from build123d import *

# Parameters (mm, degrees)
SKETCH1_W                                    = 120
SKETCH1_H                                    = 116
BOSS_EXTRUDE1_DEPTH                          = 9.525
CBORE_FOR_M4_HEX_HEAD_CAP_SCREW1_D           = 4.2
CBORE_FOR_M4_HEX_HEAD_CAP_SCREW1_CBORE_D     = 7.6
CBORE_FOR_M4_HEX_HEAD_CAP_SCREW1_CBORE_DEPTH = 4.5
SKETCH2_R                                    = 7
CUT_EXTRUDE1_DEPTH                           = 84.992414092
SKETCH5_R                                    = 1.65
CUT_EXTRUDE2_DEPTH                           = 10
SKETCH6_R                                    = 1.65
CUT_EXTRUDE3_DEPTH                           = 84.992414092
FILLET1_R                                    = 10


with BuildPart() as part:
    # Sketch1 → Boss-Extrude1 (new body)
    with BuildSketch(Plane.YZ):
        Rectangle(SKETCH1_W, SKETCH1_H)
    extrude(amount=BOSS_EXTRUDE1_DEPTH)

    # CBORE for M4 Hex Head Cap Screw1 (through all)
    with Locations(Plane(origin=(9.525, -15.556349186, 21.556349186), x_dir=(0, 0, 1), z_dir=(1, 0, 0))):
        with Locations((0, 0), (0, -31.112698372), (-31.112698372, -31.112698372), (-31.112698372, 0)):
            CounterBoreHole(CBORE_FOR_M4_HEX_HEAD_CAP_SCREW1_D / 2, CBORE_FOR_M4_HEX_HEAD_CAP_SCREW1_CBORE_D / 2, CBORE_FOR_M4_HEX_HEAD_CAP_SCREW1_CBORE_DEPTH)

    # Sketch2 → Cut-Extrude1 (cut, through all)
    with BuildSketch(Plane.YZ.offset(9.525)):
        with Locations(Location((0, 6, 0), (0, 0, 270))):
            Circle(SKETCH2_R)
    extrude(amount=-CUT_EXTRUDE1_DEPTH, mode=Mode.SUBTRACT)

    # Sketch5 → Cut-Extrude2 (cut)
    with BuildSketch(Plane(origin=(0, 0, -58), x_dir=(1, 0, 0), z_dir=(0, 0, -1))):
        with Locations(Location((4.7625, 27, 0), (0, 0, 180))):
            Circle(SKETCH5_R)
        with Locations(Location((4.7625, 0, 0), (0, 0, 180))):
            Circle(SKETCH5_R)
        with Locations(Location((4.7625, -27, 0), (0, 0, 180))):
            Circle(SKETCH5_R)
        with Locations(Location((4.7625, -54, 0), (0, 0, 180))):
            Circle(SKETCH5_R)
        with Locations(Location((4.7625, 54, 0), (0, 0, 180))):
            Circle(SKETCH5_R)
    extrude(amount=-CUT_EXTRUDE2_DEPTH, mode=Mode.SUBTRACT)

    # Sketch6 → Cut-Extrude3 (cut, through all)
    with BuildSketch(Plane.YZ.offset(9.525)):
        with Locations(Location((34, 40, 0), (0, 0, 270))):
            Circle(SKETCH6_R)
        with Locations(Location((34, -28, 0), (0, 0, 270))):
            Circle(SKETCH6_R)
        with Locations(Location((-34, -28, 0), (0, 0, 270))):
            Circle(SKETCH6_R)
        with Locations(Location((-34, 40, 0), (0, 0, 270))):
            Circle(SKETCH6_R)
    extrude(amount=-CUT_EXTRUDE3_DEPTH, mode=Mode.SUBTRACT)

    # Fillet1
    fillet1_edges = [part.edges().sort_by_distance(p)[0] for p in [
        (4.7625, -60, 58),
        (4.7625, 60, 58),
    ]]
    fillet(fillet1_edges, radius=FILLET1_R)


solid = part.part
CAD build for the part. Positions are in the model's coordinates, mm. A direction names the side the tool comes from. Give positions to 0.01 mm unless a question says otherwise; leave off trailing zeros. Loops run counter-clockwise (first coordinate to the right, second up) from the corner with the lowest first, then second, coordinate; pieces in that order, holes last. Notation, with made-up numbers: M 24.25,19 L 40.25,19 A9 cw 40.25,25 Z; hole C 71,70.5 d5. An arc over 180 degrees is marked long. Answer in a Markdown table with one row per item. Add a question column.
Item 1: Band-saw the part on A-A on y = 34. Give the cut face in (x, z) (3 decimals), then the cut area to 3 significant figures.
Item 2: Mould opens along X. For faces 1 (the face through (4.83, 56.99, 55.15)), 2 (the face through (4.977, -25.364, -53.07)), 3 (the face through (9.525, -1, 14)) say: +X half, -X half, draft (parallel to the pull), parting line (faces both ways), or undercut.
Item 3: Drop flat-ended pins along their axis: P1, Ø2, axis at x = 4.76, y = 27, coming from the -Z side; P2, Ø5.5, axis at x = 4.76, y = 54, coming from the +Z side. Give the stop position or say it passes through.
Item 4: Band-saw the part on B-B on z = -28. Give the cut face in (x, y) (3 decimals).
Item 5: Band-saw the part on C-C on y = 0. Give the cut face in (x, z) (1 decimal).
Item 6: Probe probe 1 along Y at (x, z) = (4, 6); probe 2 along Z at (x, y) = (4.5, -16); probe 3 along Y at (x, z) = (2.75, 39.5). List the from-to ranges inside material, lowest first.
Item 7: Tool access for faces 4 (the face through (4.977, 28.636, -53.07)), 5 (the face through (7.306, -13.244, 18.541)), 6 (the face through (2.477, 13.474, -9.283)): list every direction of +Z, -Z, +X, -X, +Y, -Y with a clear straight run to the whole face (end or side of a thin tool).
Item 8: Band-saw the part on D-D on y = -27. Give the cut face in (x, z) (1 decimal).
Reply:
| question | item | result |
|---|---|---|
| 1 | outline | M 0,-58 L 9.525,-58 L 9.525,-29.65 L 0,-29.65 Z; M 0,-26.35 L 9.525,-26.35 L 9.525,38.35 L 0,38.35 Z; M 0,41.65 L 9.525,41.65 L 9.525,58 L 0,58 Z |
| 1 | area | 1,040 mm^2 |
| 2 | face 1 | draft |
| 2 | face 2 | undercut |
| 2 | face 3 | +X half |
| 3 | P1 | stops at z = -48 |
| 3 | P2 | stops at z = 57.92 |
| 4 | outline | M 0,-60 L 9.525,-60 L 9.525,-35.65 L 0,-35.65 Z; M 0,-32.35 L 9.525,-32.35 L 9.525,32.35 L 0,32.35 Z; M 0,35.65 L 9.525,35.65 L 9.525,60 L 0,60 Z |
| 5 | outline | M 0,-58 L 3.1,-58 L 3.1,-48 L 6.4,-48 L 6.4,-58 L 9.5,-58 L 9.5,-1 L 0,-1 Z; M 0,13 L 9.5,13 L 9.5,58 L 0,58 Z |
| 6 | probe 1 | y = -60 to -7, 7 to 60 |
| 6 | probe 2 | z = -58 to -11.61, -7.5 to 19.5, 23.61 to 58 |
| 6 | probe 3 | y = -60 to -35.57, -32.43 to 32.43, 35.57 to 60 |
| 7 | face 4 | -Z |
| 7 | face 5 | +X |
| 7 | face 6 | +X, -X |
| 8 | outline | M 0,-58 L 3.1,-58 L 3.1,-48 L 6.4,-48 L 6.4,-58 L 9.5,-58 L 9.5,58 L 0,58 Z |
